Part model, mm, in its own coordinate system. A direction names the side the tool comes from. Coordinates: 2 decimals unless noted, no trailing zeros. Loops run counter-clockwise (first coordinate to the right, second up) from the corner with the lowest first, then second, coordinate; pieces in that order, holes last. Notation, with made-up numbers: (88, 38) -> (116, 38) arc R9 cw to (116, 43) -> close; hole circle Ø2 at (-24, -16.75). An arc over 180 degrees is marked (long way). One line per question, with ' | ' between items. Start each with the question number.
1) Probe L1, parallel to Z at x = -28.5, y = 4; L2, parallel to Z at x = -73, y = 35; L3, parallel to Y at x = -38, z = 27. List the from-to ranges inside material, lowest first. Write a range as from..to.
2) Cut at B-B (y = 21.5). Count the separate pieces of the cut face and the enclosed holes in it, plus the area to 3 significant figures.
3) Drop flat-ended pins along their axis: pin 1 (1.5 mm diameter, centred on x = -13.5, y = 1, fed in from +Z); pin 2 (12 mm diameter, centred on x = 11, z = -24, fed in from +Y); pin 3 (16.5 mm diameter, centred on x = 117, y = 12, fed in from +Z). Give the stop position or say it passes through.
4) Cut at A-A (z = -8). List the corners of the cut face in (x, y), plus the area to 3 significant figures.
5) Two-plate mould, pull along X, no slides. Class faces 1 (the face through (117, 7, -25)), 2 (the face through (-49.75, 21.5, 20.06)), 3 (the face through (-82.705, 21, 24)), 4 (the face through (137.295, 1, 0)): released by +X, released by -X, zero draft, split by the parting line, or undercut.
6) Cut at C-C (x = 31). List the corners of the cut face in (y, z), plus the area to 3 significant figures.
7) 3-axis set-ups, long thin cutter, end or side, ignore diameter. For faces 5 (the face through (117, 7, 25)), 6 (the face through (-51, 21, -35)), 7 (the face through (-50.81, 21.77, 24.71)): which of +Z, -Z, +X, -X, +Y, -Y reach the whole face in a straight line?
from build123d import *

# Parameters (mm, degrees)
SKETCH_1_W           = 220
SKETCH_1_H           = 70
EXTRUDE_1_DEPTH      = 3
EXTRUDE_2_DEPTH      = 25
EXTRUDE_2_DEPTH_BACK = 25
SKETCH_6_W           = 30
SKETCH_6_H           = 37.527767497
CUT_EXTRUDE_4_DEPTH  = 221.0000001
SKETCH_7_R           = 35
CUT_EXTRUDE_5_DEPTH  = 4
SKETCH_8_W           = 3
SKETCH_8_H           = 40
EXTRUDE_3_DEPTH      = 65
SKETCH_9_R           = 1.5
CUT_EXTRUDE_6_DEPTH  = 4
FILLET_5_R           = 1
SKETCH_10_W          = 65
SKETCH_10_H          = 20
CUT_EXTRUDE_7_DEPTH  = 4.0000001


with BuildPart() as part:
    # 草图1 → 凸台-拉伸1 (new body)
    with BuildSketch(Plane(origin=(0, 0, 0), x_dir=(1, 0, 0), z_dir=(0, 1, 0))):
        with Locations((27.295373665, 0)):
            Rectangle(SKETCH_1_W, SKETCH_1_H)
    extrude(amount=EXTRUDE_1_DEPTH)

    # 草图2 → 凸台-拉伸2 (add, two sides)
    with BuildSketch(Plane.XY) as extrude_2_sk:
        Polygon((-82.704626335, 40.527767497), (-82.704626335, 3), (-17.704626335, 3), align=None)
        with BuildLine():
            Line((137.295373665, 3), (137.295373665, 18.810437945))
            add(Edge.make_bspline(
                [(59.295373665, 3), (98.406140267, 10.357107668), (137.295373665, 18.810437945)],
                knots=[0, 0, 0, 1, 1, 1], degree=2))
            Line((59.295373665, 3), (137.295373665, 3))
        make_face()
    extrude(amount=EXTRUDE_2_DEPTH)
    extrude(extrude_2_sk.sketch, amount=-EXTRUDE_2_DEPTH_BACK)

    # 草图6 → 切除-拉伸4 (cut, through all)
    with BuildSketch(Plane.ZY.offset(82.704626335)):
        with Locations((0, 21.763883748)):
            Rectangle(SKETCH_6_W, SKETCH_6_H)
    extrude(amount=-CUT_EXTRUDE_4_DEPTH, mode=Mode.SUBTRACT)

    # 草图7 → 切除-拉伸5 (cut, through all)
    with BuildSketch(Plane(origin=(0, 3, 0), x_dir=(1, 0, 0), z_dir=(0, 1, 0))):
        with Locations((25.295373665, 51)):
            Circle(SKETCH_7_R)
        with Locations((25.295373665, -51)):
            Circle(SKETCH_7_R)
    extrude(amount=-CUT_EXTRUDE_5_DEPTH, mode=Mode.SUBTRACT)

    # 草图8 → 凸台-拉伸3 (add)
    with BuildSketch(Plane.ZY.offset(82.704626335)):
        with Locations((36.5, 20)):
            Rectangle(SKETCH_8_W, SKETCH_8_H)
        with Locations((-36.5, 20)):
            Rectangle(SKETCH_8_W, SKETCH_8_H)
    extrude(amount=-EXTRUDE_3_DEPTH)

    # 草图9 → 切除-拉伸6 (cut, through all)
    with BuildSketch(Plane(origin=(0, 3, 0), x_dir=(1, 0, 0), z_dir=(0, 1, 0))):
        with Locations((-74.766784803, 29.860059225)):
            Circle(SKETCH_9_R)
        with Locations((-54.766784803, 29.860059225)):
            Circle(SKETCH_9_R)
        with Locations((-34.766784803, 29.860059225)):
            Circle(SKETCH_9_R)
        with Locations((-34.766784803, -29.860059225)):
            Circle(SKETCH_9_R)
        with Locations((-54.766784803, -29.860059225)):
            Circle(SKETCH_9_R)
        with Locations((-74.766784803, -29.860059225)):
            Circle(SKETCH_9_R)
        with Locations((68.031562246, 29.860059225)):
            Circle(SKETCH_9_R)
        with Locations((88.031562246, 29.860059225)):
            Circle(SKETCH_9_R)
        with Locations((108.031562246, 29.860059225)):
            Circle(SKETCH_9_R)
        with Locations((108.031562246, -29.860059225)):
            Circle(SKETCH_9_R)
        with Locations((88.031562246, -29.860059225)):
            Circle(SKETCH_9_R)
        with Locations((68.031562246, -29.860059225)):
            Circle(SKETCH_9_R)
    extrude(amount=-CUT_EXTRUDE_6_DEPTH, mode=Mode.SUBTRACT)

    # 圆角5
    fillet_5_edges = [part.edges().sort_by_distance(p)[0] for p in [
        (98.35091757, 10.631195874, -25),
        (98.35091757, 10.631195874, 25),
        (-50.204626335, 21.763883749, -25),
        (-50.204626335, 21.763883749, 25),
        (-50.204626335, 21.763883749, -15),
        (-50.204626335, 21.763883749, 15),
        (98.35091757, 10.631195874, 15),
        (98.35091757, 10.631195874, -15),
    ]]
    fillet(fillet_5_edges, radius=FILLET_5_R)

    # 草图10 → 切除-拉伸7 (cut, through all)
    with BuildSketch(Plane(origin=(0, 3, 0), x_dir=(1, 0, 0), z_dir=(0, 1, 0))):
        with Locations((-50.204626335, 0)):
            Rectangle(SKETCH_10_W, SKETCH_10_H)
    extrude(amount=-CUT_EXTRUDE_7_DEPTH, mode=Mode.SUBTRACT)


solid = part.part
Reported:
1) L1: z = -38..-35, -25..-15, 15..25, 35..38 | L2: z = -38..-35, 35..38 | L3: y = 0..3
2) separate pieces: 4 | enclosed holes: 0 | area: 1,050 mm²
3) pin 1: stops at z = 35 | pin 2: stops at y = 3 | pin 3: stops at z = 25
4) outline: (-17.7, 0) -> (137.3, 0) -> (137.3, 3) -> (-17.7, 3) -> close | area: 465 mm²
5) face 1: zero draft | face 2: undercut | face 3: released by -X | face 4: released by +X
6) outline: (0, -16.47) -> (3, -16.47) -> (3, 16.47) -> (0, 16.47) -> close | area: 98.8 mm²
7) face 5: +Z, +X, -X, +Y | face 6: +X, -X, +Y | face 7: +Y
